For this review, take the finished solid that the model builds, in its own axes (mm). A direction names the side the tool comes from. Round coordinates to 2 decimals unless told otherwise and drop trailing zeros. Order: outer loops, then holes, each group sorted by start corner. A loop starts at its lowest first (then second) coordinate and runs counter-clockwise, first axis right, second up. Notation, with made-up numbers: M 38,3 L 70,3 A29 cw 70,25 Z; hole C -18.5,62.5 d5. An arc over 180 degrees is marked long. Answer as a JSON object with one key per item and string values.
from build123d import *

# Parameters (mm, degrees)
EXTRUDE001_DEPTH           = 1
EXTRUDE_DEPTH              = 1
TUBE_R                     = 6
TUBE_R_2                   = 5
TUBE_DEPTH                 = 1
EXTRUDE002_DEPTH           = 1
EXTRUDE002_PLACEMENT_ANGLE = 180


with BuildPart() as extrude001:
    # Sketch → Extrude001 (new body)
    with BuildSketch(Plane.XY):
        with BuildLine():
            ThreePointArc((-5.554538, 7.282242), (-6.309564, 5.15544), (-4.995944, 3.320296))
            Line((-4.995944, 3.320296), (-4.163386, 3.976998))
            ThreePointArc((-5.554538, 7.282242), (-5.403982, 5.400225), (-4.163386, 3.976998))
        make_face()
    extrude(amount=EXTRUDE001_DEPTH)


with BuildPart() as extrude_body:
    # Sketch → Extrude (new body)
    with BuildSketch(Plane.XY):
        with BuildLine():
            ThreePointArc((-5.554538, 7.282242), (-6.309564, 5.15544), (-4.995944, 3.320296))
            Line((-4.995944, 3.320296), (-4.163386, 3.976998))
            ThreePointArc((-5.554538, 7.282242), (-5.403982, 5.400225), (-4.163386, 3.976998))
        make_face()
    extrude(amount=EXTRUDE_DEPTH)


with BuildPart() as tube:
    # Tube → Tube (new body)
    with BuildSketch(Plane(origin=(-1, 0, 0), x_dir=(1, 0, 0), z_dir=(0, 0, 1))):
        Circle(TUBE_R)
        Circle(TUBE_R_2, mode=Mode.SUBTRACT)
    extrude(amount=TUBE_DEPTH)


with BuildPart() as fusion:
    # Sketch001 → Extrude002 (new body)
    with BuildSketch(Plane.XY):
        with BuildLine():
            ThreePointArc((-5.554538, 7.282242), (-6.309564, 5.15544), (-4.995944, 3.320296))
            Line((-4.995944, 3.320296), (-4.163386, 3.976998))
            ThreePointArc((-5.554538, 7.282242), (-5.403982, 5.400225), (-4.163386, 3.976998))
        make_face()
    extrude(amount=EXTRUDE002_DEPTH)


with BuildPart() as fusion_1:
    # Extrude002 placement: moved
    add(fusion.part.moved(Location((-1.914214, 0, 0.914214))).rotate(Axis((-1.914214, 0, 0.914214), (0, 1, 0)), EXTRUDE002_PLACEMENT_ANGLE))

    # Fusion: union Extrude001, Extrude body, Tube
    add(extrude001.part)
    add(extrude_body.part)
    add(tube.part)


solid = fusion_1.part
1) Add section D-D on y = 5.75. State the section outline as (x, z) points, and give its area (3 significant figures).
Geometry check:
{"outline": "M -6.32,0 L -5.53,0 L -5.53,1 L -6.32,1 Z; M -2.71,0 L 0.71,0 L 0.71,1 L -2.71,1 Z; M 3.61,-0.09 L 4.41,-0.09 L 4.41,0.91 L 3.61,0.91 Z", "area": "5.02 mm²"}
2) Add section C-C on z = 0.5. State the section outline as (x, y) points (1 decimal), and give its area (3 significant figures).
Geometry check:
{"outline": "M -5.6,3.8 A6 ccw long 3.7,3.8 A2.4 ccw 3.6,7.3 A3 cw 2.9,4.5 A6 ccw -4.9,4.6 A3 cw -5.6,7.3 A2.4 ccw Z; hole C -1,0 d10", "area": "39.4 mm²"}
3) For L1, parallel to Y at x = -1, z = 0.5; L2, parallel to Z at x = 4.5, y = -1; L3, parallel to X at y = 0.5, z = 0.4, list the stretches that pass through material, from the lowest coordinate up.
Geometry check:
{"L1": "y = -6 to -5, 5 to 6", "L2": "z = 0 to 1", "L3": "x = -6.98 to -5.97, 3.97 to 4.98"}
4) Machinability: for faces 1 (the flat face through (4, 5, -0.086)), 2 (the flat face through (4, 5, 0.914)), 3 (the cylindrical face through (-5.557, 5.865, 0.493)), which of the approach directions +Z, -Z, +X, -X, +Y, -Y give a long, thin tool a straight path to every point of the face, cutting with its end or side? Answer none if there is none.
Geometry check:
{"face 1": "-Z, +X, -X, +Y, -Y", "face 2": "+Z, +X, +Y", "face 3": "+Z, -Z"}
5) Mouldability with a two-part tool opening along X and no side actions: class faces 4 (the cylindrical face through (-6.33, 5.59, 0.49)), 5 (the cylindrical face through (3.1, -4.38, 0.49)), 6 (the flat face through (-4.14, 4.12, 1)) as +X half, -X half, draft (parallel to the pull), parting line (faces both ways), or undercut.
Geometry check:
{"face 4": "-X half", "face 5": "undercut", "face 6": "draft"}
6) Insertion check: P1, Ø1.5, axis at x = -2.5, y = 3.5, coming from the -Z side; P2, Ø3.5, axis at x = -3.5, y = 3, coming from the -Z side. Each pin has a flat end and moves straight along its axis. Give the tip position at first contact, or say it passes through.
Geometry check:
{"P1": "passes through", "P2": "stops at z = 0"}
7) Add section A-A on y = 0. State the section outline as (x, z) points.
Geometry check:
{"outline": "M -7,0 L -6,0 L -6,1 L -7,1 Z; M 4,0 L 5,0 L 5,1 L 4,1 Z"}
8) Add section B-B on x = -1. State the section outline as (y, z) points.
Geometry check:
{"outline": "M -6,0 L -5,0 L -5,1 L -6,1 Z; M 5,0 L 6,0 L 6,1 L 5,1 Z"}
